Input: part model. Units: mm. Frame: model coordinates. Face numbers are marked on the shaded views. A direction names the side the tool comes from. Round coordinates to 2 decimals unless told otherwise and drop trailing zeros. Loops run counter-clockwise (first coordinate to the right, second up) from the corner with the lowest first, then second, coordinate; pieces in that order, holes last. Notation, with made-up numbers: (6.25, 10) -> (21.25, 10) arc R18 cw to (21.25, 24) -> close; hole circle Ø10 at (-29, 55). An arc over 180 degrees is marked (long way). Answer as a JSON object with one key per item and string values. Group by question number.
Item 1: Section query A-A on y = 88.9. Return loops of the section in (x, z) (3 decimals).
Item 2: Section query D-D on y = 63.5. Return loops of the section in (x, z) (3 decimals), and give its area (3 significant figures).
Item 3: Set-up query: the marked faces 1, 2 and 3. Return all of +Z, -Z, +X, -X, +Y, -Y with unobstructed straight access to the full face (end or side cutting, diameter ignored); none if empty.
Item 4: Section query B-B on x = 114.3. Return loops of the section in (y, z) (1 decimal), and give its area (3 significant figures).
Item 5: Pin query (flat end, axial travel): pin 1 (4.5 mm diameter, centred on x = 12.7, y = 88.9, fed in from +Z); pin 2 (6.5 mm diameter, centred on x = 25.4, y = 50.8, fed in from +Z) (3 decimals). Return the tip coordinate at first contact, or that it passes through.
Item 6: Section query C-C on y = -56. Return loops of the section in (x, z) (3 decimals), and give its area (3 significant figures).
Item 7: Material intervals for line 1 (X direction, y = 88, z = 2); line 2 (X direction, y = 75, z = 12); line 3 (Z direction, x = 34, y = 43.5) (3 decimals), sorted ascending. Write a range as [from, to].
from build123d import *

# Parameters (mm, degrees)
SKETCH1_R           = 2.4892
SKETCH1_R_2         = 14.2875
BOSS_EXTRUDE1_DEPTH = 3.175
JOG1_START          = -71.4375
JOG1_DEPTH          = 173.0375
JOG1_2_DEPTH        = 101.6
JOG1_START_2        = -36.5124999
JOG1_3_OUTLINE_W    = 63.5
JOG1_3_OUTLINE_H    = 3.175
JOG1_3_DEPTH        = 11.1124999
JOG1_START_3        = 114.3
JOG1_4_OUTLINE_R    = 14.2875
JOG1_4_DEPTH        = 3.175
FILLET2_R           = 6.35


with BuildPart() as part:
    # Sketch1 → Boss-Extrude1 (new body)
    with BuildSketch(Plane.XY):
        Polygon((0, 0), (82.55, 0), (82.55, -50.8), (105.480555556, -71.4375), (123.119444444, -71.4375), (146.05, -50.8), (146.05, -25.4), (107.95, 101.6), (0, 101.6), align=None)
        with Locations((12.7, 12.7)):
            Circle(SKETCH1_R, mode=Mode.SUBTRACT)
        with Locations((25.4, 12.7)):
            Circle(SKETCH1_R, mode=Mode.SUBTRACT)
        with Locations((38.1, 12.7)):
            Circle(SKETCH1_R, mode=Mode.SUBTRACT)
        with Locations((12.7, 25.4)):
            Circle(SKETCH1_R, mode=Mode.SUBTRACT)
        with Locations((25.4, 25.4)):
            Circle(SKETCH1_R, mode=Mode.SUBTRACT)
        with Locations((12.7, 38.1)):
            Circle(SKETCH1_R, mode=Mode.SUBTRACT)
        with Locations((12.7, 50.8)):
            Circle(SKETCH1_R, mode=Mode.SUBTRACT)
        with Locations((25.4, 38.1)):
            Circle(SKETCH1_R, mode=Mode.SUBTRACT)
        with Locations((25.4, 50.8)):
            Circle(SKETCH1_R, mode=Mode.SUBTRACT)
        with Locations((38.1, 25.4)):
            Circle(SKETCH1_R, mode=Mode.SUBTRACT)
        with Locations((38.1, 38.1)):
            Circle(SKETCH1_R, mode=Mode.SUBTRACT)
        with Locations((38.1, 50.8)):
            Circle(SKETCH1_R, mode=Mode.SUBTRACT)
        with Locations((12.7, 63.5)):
            Circle(SKETCH1_R, mode=Mode.SUBTRACT)
        with Locations((12.7, 76.2)):
            Circle(SKETCH1_R, mode=Mode.SUBTRACT)
        with Locations((25.4, 63.5)):
            Circle(SKETCH1_R, mode=Mode.SUBTRACT)
        with Locations((25.4, 76.2)):
            Circle(SKETCH1_R, mode=Mode.SUBTRACT)
        with Locations((12.7, 88.9)):
            Circle(SKETCH1_R, mode=Mode.SUBTRACT)
        with Locations((25.4, 88.9)):
            Circle(SKETCH1_R, mode=Mode.SUBTRACT)
        with Locations((38.1, 63.5)):
            Circle(SKETCH1_R, mode=Mode.SUBTRACT)
        with Locations((38.1, 76.2)):
            Circle(SKETCH1_R, mode=Mode.SUBTRACT)
        with Locations((38.1, 88.9)):
            Circle(SKETCH1_R, mode=Mode.SUBTRACT)
        with Locations((114.3, -50.8)):
            Circle(SKETCH1_R_2, mode=Mode.SUBTRACT)
    extrude(amount=BOSS_EXTRUDE1_DEPTH)

    # Jog1: read off the stored shape, not the designer's step
    # Jog1 outline → Jog1 (cut)
    with BuildSketch(Plane(origin=(0, 0, 0), x_dir=(1, 0, 0), z_dir=(0, 1, 0)).offset(JOG1_START)):
        with BuildLine():
            ThreePointArc((72.459541247, 0), (75.634541247, -0.850738686), (77.958802561, -3.175))
            Line((77.958802561, -3.175), (146.05, -3.175))
            Line((146.05, -3.175), (146.05, 0))
            Line((146.05, 0), (72.459541247, 0))
        make_face()
    extrude(amount=JOG1_DEPTH, mode=Mode.SUBTRACT)

    # Jog1 2 outline → Jog1 2 (add)
    with BuildSketch(Plane(origin=(0, 0, 0), x_dir=(1, 0, 0), z_dir=(0, 1, 0))):
        with BuildLine():
            ThreePointArc((72.459541247, -3.175), (74.704605277, -4.10493597), (75.634541247, -6.35))
            Line((75.634541247, -6.35), (75.634541247, -111.125))
            ThreePointArc((75.634541247, -111.125), (77.494413186, -115.615128061), (81.984541247, -117.475))
            Line((81.984541247, -117.475), (82.55, -117.475))
            Line((82.55, -117.475), (82.55, -114.3))
            Line((82.55, -114.3), (81.984541247, -114.3))
            ThreePointArc((81.984541247, -114.3), (79.739477217, -113.37006403), (78.809541247, -111.125))
            Line((78.809541247, -111.125), (78.809541247, -6.35))
            ThreePointArc((78.809541247, -6.35), (78.593170244, -4.706499064), (77.958802561, -3.175))
            Line((77.958802561, -3.175), (72.459541247, -3.175))
        make_face()
    extrude(amount=JOG1_2_DEPTH)



with BuildPart() as body_2:
    # Jog1 3 outline → Jog1 3 (new body)
    with BuildSketch(Plane(origin=(0, 0, 0), x_dir=(1, 0, 0), z_dir=(0, 1, 0)).offset(JOG1_START_2)):
        with Locations((114.3, -115.8875)):
            Rectangle(JOG1_3_OUTLINE_W, JOG1_3_OUTLINE_H)
    extrude(amount=JOG1_3_DEPTH)


with BuildPart() as part_1:
    add(part.part)

    add(body_2.part)  # Jog1 4 merges body 2
    # Jog1 4 outline → Jog1 4 (add)
    with BuildSketch(Plane.XY.offset(JOG1_START_3)):
        Polygon((107.95, 101.6), (81.984541247, 101.6), (81.984541247, 0), (82.55, 0), (82.55, -50.8), (105.480555556, -71.4375), (123.119444444, -71.4375), (146.05, -50.8), (146.05, -25.4), align=None)
        with Locations((114.3, -50.8)):
            Circle(JOG1_4_OUTLINE_R, mode=Mode.SUBTRACT)
    extrude(amount=JOG1_4_DEPTH)

    # Fillet2
    fillet2_edges = [part_1.edges().sort_by_distance(p)[0] for p in [
        (0, 0, 1.5875),
        (0, 101.6, 1.5875),
        (107.95, 101.6, 115.8875),
        (146.05, -25.4, 115.8875),
        (146.05, -50.8, 115.8875),
        (123.119444444, -71.4375, 115.8875),
        (105.480555556, -71.4375, 115.8875),
        (82.55, -50.8, 115.8875),
    ]]
    fillet(fillet2_edges, radius=FILLET2_R)


solid = part_1.part
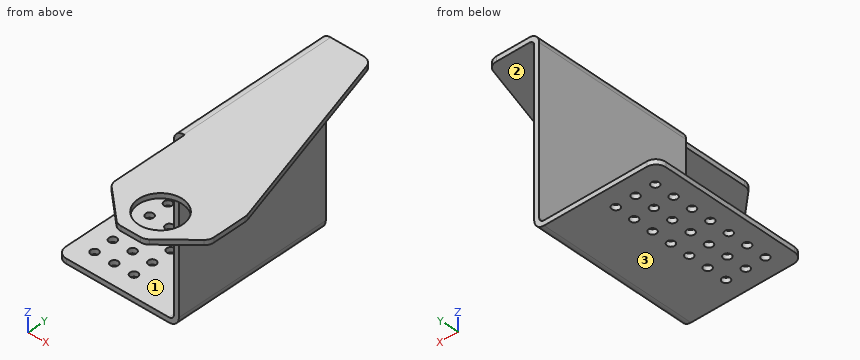
Solved:
{
 "1": {"outline": "(0, 0) -> (10.211, 0) -> (10.211, 3.175) -> (0, 3.175) -> close; (15.189, 0) -> (22.911, 0) -> (22.911, 3.175) -> (15.189, 3.175) -> close; (27.889, 0) -> (35.611, 0) -> (35.611, 3.175) -> (27.889, 3.175) -> close; (40.589, 0) -> (72.46, 0) arc R6.35 ccw to (78.81, 6.35) -> (78.81, 111.125) arc R3.175 cw to (81.985, 114.3) -> (111.76, 114.3) -> (111.76, 117.475) -> (81.985, 117.475) arc R6.35 ccw to (75.635, 111.125) -> (75.635, 6.35) arc R3.175 cw to (72.46, 3.175) -> (40.589, 3.175) -> close"},
 "2": {"outline": "(0, 0) -> (10.211, 0) -> (10.211, 3.175) -> (0, 3.175) -> close; (15.189, 0) -> (22.911, 0) -> (22.911, 3.175) -> (15.189, 3.175) -> close; (27.889, 0) -> (35.611, 0) -> (35.611, 3.175) -> (27.889, 3.175) -> close; (40.589, 0) -> (72.46, 0) arc R6.35 ccw to (78.81, 6.35) -> (78.81, 111.125) arc R3.175 cw to (81.985, 114.3) -> (119.38, 114.3) -> (119.38, 117.475) -> (81.985, 117.475) arc R6.35 ccw to (75.635, 111.125) -> (75.635, 6.35) arc R3.175 cw to (72.46, 3.175) -> (40.589, 3.175) -> close", "area": "682 mm²"},
 "3": {"face 1": "+Z, -X, +Y, -Y", "face 2": "-Z, +X, +Y, -Y", "face 3": "-Z, +X, -X, +Y, -Y"},
 "4": {"outline": "(-71.4, 114.3) -> (-65.1, 114.3) -> (-65.1, 117.5) -> (-71.4, 117.5) -> close; (-36.5, 114.3) -> (80.4, 114.3) -> (80.4, 117.5) -> (-36.5, 117.5) -> close", "area": "391 mm²"},
 "5": {"pin 1": "through", "pin 2": "z = 3.175"},
 "6": {"outline": "(88.328, 114.3) -> (100.992, 114.3) -> (100.992, 117.475) -> (88.328, 117.475) -> close; (127.608, 114.3) -> (140.272, 114.3) -> (140.272, 117.475) -> (127.608, 117.475) -> close", "area": "80.4 mm²"},
 "7": {"line 1": "[0, 10.38], [15.02, 23.08], [27.72, 35.78], [40.42, 77.09]", "line 2": "[75.63, 78.81]", "line 3": "[0, 3.175]"}
}
